Could you check a few things on this model? Use its own coordinates, in mm. Round coordinates to 2 decimals unless told otherwise and drop trailing zeros. Write each loop counter-clockwise with the first axis right and the second up, starting at its lowest first coordinate (ties: lowest second). Pieces come first, ordered by that corner, then holes. Notation, with made-up numbers: (50, 53) -> (97, 53) arc R27 ccw to (97, 88) -> close; hole circle Ø11 at (78, 50). An arc over 180 degrees is marked (long way). One line per question, with ' | ' between items. Start each with the question number.
1. For pin 1 Ø8 at (y, z) = (-15, 113) entering from +X, with a flat end and sliding along its axis, tell me the tip position at first contact or that it passes through.
2. Imagine slicing it at B-B, the plane z = 248. List the corners of the cut face in (x, y) for me, and give its area (3 significant figures).
3. Imagine slicing it at C-C, the plane y = -5. List the corners of the cut face in (x, z) for me, and give its area (3 significant figures).
4. Imagine slicing it at A-A, the plane x = 33. List the corners of the cut face in (y, z) for me.
5. If I drill on line 1 along X through (y, z) = (-21, 509); line 2 along Y through (x, z) = (12.5, 614); line 3 along Y through (x, z) = (11, 409.5), over which ranges is the centre line in solid material (lowest first)? Write a range as [from, to].
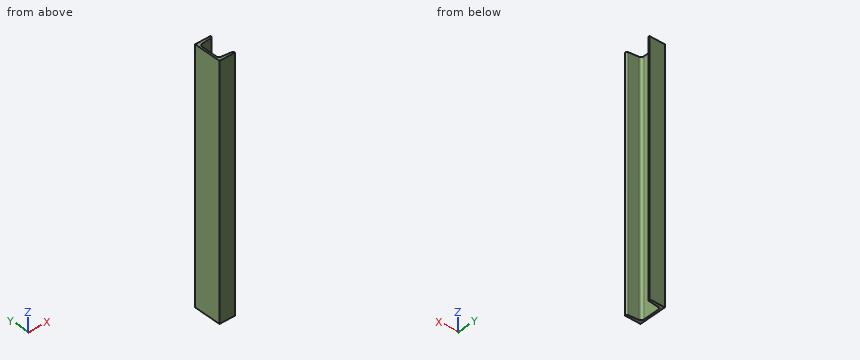
Autodesk Inventor part; units mm, degrees
ref_plane "Начальная плоскость" through (0, 0, 0) normal (0, 0, 1) x (1, 0, 0)
ref_plane "Конечная плоскость" through (0, 0, 720.5) normal (0, 0, 1) x (1, 0, 0)
ref_plane "YZ Plane" through (0, 0, 0) normal (1, 0, 0) x (0, 1, 0)
ref_plane "Начальная плоскость" through (0, 0, 0) normal (0, 0, 1) x (1, 0, 0)
ref_plane "Конечная плоскость" through (0, 0, 720.5) normal (0, 0, 1) x (1, 0, 0)
sketch "Эскиз" plane through (0, 0, 0) normal (0, 0, 1) x (1, 0, 0)
  line L0 (-1.43, 0) -> (-1.43, 40)
  line L1 (-1.43, 40) -> (43.57, 40)
  line L2 (43.57, 40) -> (43.57, 38.1774)
  line L3 (39.9881, 34.1993) -> (11.2338, 31.1771)
  line L4 (4.07, 23.221) -> (4.07, 0)
  line L5 (4.07, 0) -> (-1.43, 0) construction
  line L6 (23.82, 40) -> (23.82, 32.5) construction
  line L7 (43.57, 34.5758) -> (43.57, 32.5) construction
  line L8 (43.57, 32.5) -> (23.82, 32.5) construction
  line L9 (0, 15) -> (0, -27) construction
  line L10 (-5.539, 0) -> (16.0067, 0) construction
  line L11 (-1.43, 0) -> (-1.43, -40)
  line L12 (-1.43, -40) -> (43.57, -40)
  line L13 (43.57, -40) -> (43.57, -38.1774)
  line L14 (39.9881, -34.1993) -> (11.2338, -31.1771)
  line L15 (4.07, -23.221) -> (4.07, 0)
  arc A0 (11.2338, 31.1771) -> (4.07, 23.221) centre (12.07, 23.221) ccw
  arc A1 (4.07, -23.221) -> (11.2338, -31.1771) centre (12.07, -23.221) ccw
  arc A2 (39.9881, 34.1993) -> (43.57, 38.1774) centre (39.57, 38.1774) ccw
  arc A3 (43.57, -38.1774) -> (39.9881, -34.1993) centre (39.57, -38.1774) ccw
  line L16 (0, 56) -> (0, -56) construction
  line L17 (-15.5135, 0) -> (54.308, 0) construction
  point P0 (4.07, 30.4242)
  point P1 (43.57, -34.5758)
  point P2 (4.07, -30.4242)
  point P3 (23.82, -40)
  point P4 (23.82, -32.5)
  dimension "d0" = 5.5
  dimension "d1" = 40
  dimension "d2" = 45
  dimension "d3" = 7.5
  dimension "d4" = 19.75
  dimension "d5" = 2.0758
  dimension "d23" = 8
  dimension "d24" = 4
  dimension "d25" = 1.43
extrude "Тело" add sketch "Эскиз" along normal up to surface (720.5 mm away) from surface at 0
sketch "Sketch3" plane through (0, 0, 0) normal (0, 0, 1) x (1, 0, 0)
  line L0 (0, 0) -> (10, 0)
ref_plane "Work Plane3" through (0, 0, 0) normal (0, -1, 0) x (1, 0, 0)
sketch "Sketch4" plane through (0, 0, 0) normal (0, -1, 0) x (1, 0, 0)
  line L0 (-2, 0) -> (12, 0)
  line L1 (-2, 720.5) -> (12, 720.5)
  dimension "d29" = 720.5
equation "\"d0\" = G_T"
equation "\"d1\" = 0.5 * G_H"
equation "\"d2\" = G_W"
equation "\"d3\" = G_T1"
equation "\"d4\" = G_C"
equation "\"d23\" = G_IR"
equation "\"d24\" = G_ER"
equation "\"d25\" = ex"
equation "\"d6\" = G_L"
equation "\"G_W\" = 45"
equation "\"G_T\" = 5.5"
equation "\"G_T1\" = 7.5"
equation "\"G_NG\" = 0.105104"
equation "\"G_ER\" = 4"
equation "\"G_IR\" = 8"
equation "\"G_C\" = 19.75"
equation "\"G_L\" = d29"
equation "\"ex\" = 1.43"
equation "\"G_OFFSET_START\" = 0"
equation "\"G_OFFSET_END\" = 0"
equation "\"d27\" = G_OFFSET_END + B_L"
equation "\"B_L\" = 720.5"
properties part number "ISO 657/11 - CH 80 x 8 - 720,5" material "Сталь, мягкая"
Geometry results:
1) pin 1: stops at x = 4.07
2) outline: (-1.43, -40) -> (43.57, -40) -> (43.57, -38.18) arc R4 ccw to (39.99, -34.2) -> (11.23, -31.18) arc R8 cw to (4.07, -23.22) -> (4.07, 23.22) arc R8 cw to (11.23, 31.18) -> (39.99, 34.2) arc R4 ccw to (43.57, 38.18) -> (43.57, 40) -> (-1.43, 40) -> close | area: 1,050 mm2
3) outline: (-1.43, 0) -> (4.07, 0) -> (4.07, 720.5) -> (-1.43, 720.5) -> close | area: 3,960 mm2
4) outline: (-40, 0) -> (-33.46, 0) -> (-33.46, 720.5) -> (-40, 720.5) -> close; (33.46, 0) -> (40, 0) -> (40, 720.5) -> (33.46, 720.5) -> close
5) line 1: x = [-1.43, 4.07] | line 2: y = [-40, -31.31], [31.31, 40] | line 3: y = [-40, -31.15], [31.15, 40]
